from build123d import *

# Parameters (mm, degrees)
F1_DEPTH = 60
F3_DEPTH = 15
F4_R     = 5
F5_DEPTH = 15
F7_DEPTH = 30.0010001
F8_R     = 25
F9_DEPTH = 60.0010001


# Not quite as in the source:
# - a pattern or mirror of a feature is missing from the dataset's text; its kind, count and spacing are read off the source's solid


with BuildPart() as f1:
    # F0 (on Front) → F1 (new body)
    with BuildSketch(Plane.XZ):
        with BuildLine():
            Line((-30, 0), (30, 0))
            ThreePointArc((30, 0), (0, 30), (-30, 0))
        make_face()
    extrude(amount=-F1_DEPTH)

    # F2 (on Top) → F3 (join)
    with BuildSketch(Plane.XY):
        with BuildLine():
            ThreePointArc((-40, 60), (-50, 50), (-40, 40))
            Line((-40, 40), (40, 40))
            ThreePointArc((40, 40), (50, 50), (40, 60))
            Line((40, 60), (-40, 60))
        make_face()
    extrude(amount=F3_DEPTH)

    # F4 (on Top) → F5 (cut, through all)
    with BuildSketch(Plane.XY):
        with Locations((-40, 50)):
            Circle(F4_R)
    f5 = extrude(amount=F5_DEPTH, mode=Mode.SUBTRACT)

    # F5_copies: F5 across plane
    add(f5.mirror(Plane(origin=(0, 0, 0), x_dir=(0, 0, 1), z_dir=(1, 0, 0))), mode=Mode.SUBTRACT)

    # F6 (on Top) → F7 (cut, through all)
    with BuildSketch(Plane.XY):
        with BuildLine():
            Line((-10, 20), (-10, 0))
            Line((-10, 0), (0, 0))
            Line((0, 0), (0, 30))
            ThreePointArc((0, 30), (-7.0710678119, 27.0710678119), (-10, 20))
        make_face()
        with BuildLine():
            Line((0, 30), (0, 0))
            Line((0, 0), (10, 0))
            Line((10, 0), (10, 20))
            ThreePointArc((10, 20), (7.0710678119, 27.0710678119), (0, 30))
        make_face()
    extrude(amount=F7_DEPTH, mode=Mode.SUBTRACT)

    # F8 (on face) → F9 (cut, through all)
    with BuildSketch(Plane.XZ):
        Circle(F8_R)
    extrude(amount=-F9_DEPTH, mode=Mode.SUBTRACT)


solid = f1.part
Verification items for the finished model (mm, model axes). A direction names the side the tool comes from. Round coordinates to 2 decimals unless told otherwise and drop trailing zeros. Loops run counter-clockwise (first coordinate to the right, second up) from the corner with the lowest first, then second, coordinate; pieces in that order, holes last. Notation, with made-up numbers: (-8, 35) - (42, 35) arc R15 ccw to (42, 47) - close; hole circle Ø7 at (-12, -39.75). An arc over 180 degrees is marked (long way). Use a Markdown table: item, result. Add a question column.
1. Access from +Z, -Z, +X, -X, +Y, -Y to the whole of each face (thin tool, end or side, straight path). Record for faces 4 (the face through (-35, 52, 15)), 5 (the face through (-10, 10, 26)), 6 (the face through (-9.64, 29.58, 28.41)).
2. Section check A-A, the plane y = 50. Record the boundary of the cut face in (x, z).
3. Thickness scan on probe 1 along Y at (x, z) = (-40, 4); probe 2 along Z at (x, y) = (-35.5, 58); probe 3 along X at (y, z) = (22.5, 5). Record the ranges inside material, lowest first. Write a range as [from, to].
4. Gauge pin test, flat ends, axial feed: pin 1 (6 mm diameter, centred on y = 11.5, z = 26, fed in from -X); pin 2 (3 mm diameter, centred on y = 49.5, z = 18, fed in from -X); pin 3 (5 mm diameter, centred on y = 28, z = 12, fed in from -X). Record the tip position at first contact, or that the pin passes through.
5. Section check D-D, the plane y = 36. Record the boundary of the cut face in (x, z), plus the area to 3 significant figures.
6. Section check B-B, the plane z = 6. Record the boundary of the cut face in (x, y), plus the area to 3 significant figures.
7. Release check for a two-part mould opening along Z. For faces 1 (the face through (34, 40, 7)), 2 (the face through (-32, 44, 0)), 3 (the face through (35, 52, 15)) record: released by +Z, released by -Z, zero draft, split by the parting line, or undercut.
8. Section check C-C, the plane z = 24. Record the boundary of the cut face in (x, y).
Checks:
| question | item | result |
|---|---|---|
| 1 | face 4 | +Z, -X, +Y, -Y |
| 1 | face 5 | +Z, -Z, -Y |
| 1 | face 6 | +Z, -Y |
| 2 | outline | (-50, 0) - (-45, 0) - (-45, 15) - (-50, 15) - close; (-35, 0) - (-25, 0) arc R25 cw to (25, 0) - (35, 0) - (35, 15) - (25.98, 15) arc R30 ccw to (-25.98, 15) - (-35, 15) - close; (45, 0) - (50, 0) - (50, 15) - (45, 15) - close |
| 3 | probe 1 | y = [40, 45], [55, 60] |
| 3 | probe 2 | z = [0, 15] |
| 3 | probe 3 | x = [-29.58, -24.49], [24.49, 29.58] |
| 4 | pin 1 | stops at x = -19.26 |
| 4 | pin 2 | stops at x = -25.05 |
| 4 | pin 3 | stops at x = -28.46 |
| 5 | outline | (-30, 0) - (-25, 0) arc R25 cw to (25, 0) - (30, 0) arc R30 ccw to start |
| 5 | area | 432 mm^2 |
| 6 | outline | (-40, 40) - (-29.39, 40) - (-29.39, 0) - (-24.27, 0) - (-24.27, 60) - (-40, 60) arc R10 ccw to start; (24.27, 0) - (29.39, 0) - (29.39, 40) - (40, 40) arc R10 ccw to (40, 60) - (24.27, 60) - close; hole circle Ø10 at (-40, 50); hole circle Ø10 at (40, 50) |
| 6 | area | 1,200 mm^2 |
| 7 | face 1 | zero draft |
| 7 | face 2 | released by -Z |
| 7 | face 3 | released by +Z |
| 8 | outline | (-18, 0) - (-10, 0) - (-10, 20) arc R10 cw to (-7, 27.14) - (-7, 60) - (-18, 60) - close; (7, 27.14) arc R10 cw to (10, 20) - (10, 0) - (18, 0) - (18, 60) - (7, 60) - close |
